```python
from build123d import *

# Parameters (mm, degrees)
SKETCH_W     = 500
SKETCH_H     = 390
PAD_DEPTH    = 18
SKETCH001_W  = 9
SKETCH001_H  = 390
POCKET_DEPTH = 9


with BuildPart() as part:
    # Sketch → Pad (new body)
    with BuildSketch(Plane.XY):
        with Locations((-250, 195)):
            Rectangle(SKETCH_W, SKETCH_H)
    extrude(amount=PAD_DEPTH)

    # Sketch001 → Pocket (cut)
    with BuildSketch(Plane.XY):
        with Locations((-4.5, 195)):
            Rectangle(SKETCH001_W, SKETCH001_H)
        with Locations((-495.5, 195)):
            Rectangle(SKETCH001_W, SKETCH001_H)
    extrude(amount=POCKET_DEPTH, mode=Mode.SUBTRACT)


solid = part.part
```
Source: CAD feature listing. Evaluate the final solid. Frame: model axes, mm. Give positions to 0.01 mm unless a question says otherwise; leave off trailing zeros. Loops run counter-clockwise (first coordinate to the right, second up) from the corner with the lowest first, then second, coordinate; pieces in that order, holes last. Notation, with made-up numbers: (-32.5, 67.5) -> (16.5, 67.5) arc R25 ccw to (16.5, 80.5) -> close; hole circle Ø7 at (87, -35.5). An arc over 180 degrees is marked (long way). Use a Markdown table: item, result. Add a question column.
(1) Ray query, line 1 (X direction, y = 124, z = 7). Return the intervals inside material, ascending.
(2) Section query B-B (z = 6.25). Output: boundary loops of the cut face in (x, y), then the cut area to 3 significant figures.
(3) Section query A-A (y = 309). Output: boundary loops of the cut face in (x, z).
(4) First-contact query: pin 1 Ø2.5 at (x, y) = (-495.5, 215.5) entering from -Z; pin 2 Ø2.5 at (y, z) = (277, 4.5) entering from -X; pin 3 Ø7 at (y, z) = (133, 5) entering from +X. Flat tips, straight axial feed; report the tip coordinate or a pass-through.
Checked values:
| question | item | result |
|---|---|---|
| 1 | line 1 | -491 to -9 |
| 2 | outline | (-491, 0) -> (-9, 0) -> (-9, 390) -> (-491, 390) -> close |
| 2 | area | 188,000 mm^2 |
| 3 | outline | (-500, 9) -> (-491, 9) -> (-491, 0) -> (-9, 0) -> (-9, 9) -> (0, 9) -> (0, 18) -> (-500, 18) -> close |
| 4 | pin 1 | z = 9 |
| 4 | pin 2 | x = -491 |
| 4 | pin 3 | x = -9 |
